Build history of the part. All positions in model axes, mm. Round coordinates to 2 decimals unless told otherwise and drop trailing zeros. Loops run counter-clockwise (first coordinate to the right, second up) from the corner with the lowest first, then second, coordinate; pieces in that order, holes last. Notation, with made-up numbers: (19.25, 83.25) - (54.25, 83.25) arc R13 cw to (54.25, 99.25) - close; hole circle Ø2 at (24.25, 19.5). An arc over 180 degrees is marked (long way). Put each result on its own line as item: value. Start each with the question number.
from build123d import *

# Parameters (mm, degrees)
SKETCH1_W           = 152.4
SKETCH1_H           = 241.3
BOSS_EXTRUDE1_DEPTH = 3.175
SKETCH2_W           = 3.429
SKETCH2_H           = 168.148
SKETCH2_H_2         = 40.386
CUT_EXTRUDE1_DEPTH  = 286.414664348
SKETCH3_W           = 119.38
SKETCH3_H           = 119.38
SKETCH3_W_2         = 74.6125
SKETCH3_H_2         = 25.4
SKETCH3_W_3         = 12.7
SKETCH3_H_3         = 16.256
SKETCH3_W_4         = 5.334
SKETCH3_H_4         = 7.239
CUT_EXTRUDE2_DEPTH  = 286.414664348
SKETCH4_W           = 184.697558878
SKETCH4_H           = 63.754
CUT_EXTRUDE5_DEPTH  = 286.414664348
SKETCH5_W           = 3.429
SKETCH5_H           = 11.43
BOSS_EXTRUDE2_DEPTH = 3.175


with BuildPart() as part:
    # Sketch1 → Boss-Extrude1 (new body)
    with BuildSketch(Plane.XY):
        with Locations((76.2, 120.65)):
            Rectangle(SKETCH1_W, SKETCH1_H)
    extrude(amount=BOSS_EXTRUDE1_DEPTH)

    # Sketch2 → Cut-Extrude1 (cut, through all)
    with BuildSketch(Plane.XY.offset(3.175)):
        with Locations((150.6855, 139.065)):
            Rectangle(SKETCH2_W, SKETCH2_H)
        with Locations((1.7145, 139.065)):
            Rectangle(SKETCH2_W, SKETCH2_H)
        with Locations((150.6855, 20.193)):
            Rectangle(SKETCH2_W, SKETCH2_H_2)
        with Locations((1.7145, 20.193)):
            Rectangle(SKETCH2_W, SKETCH2_H_2)
    extrude(amount=-CUT_EXTRUDE1_DEPTH, mode=Mode.SUBTRACT)

    # Sketch3 → Cut-Extrude2 (cut, through all)
    with BuildSketch(Plane.XY.offset(3.175)):
        Polygon((128.016, 57.15), (140.716, 57.15), (140.716, 44.45), align=None)
        Polygon((125.77093597, 42.20493597), (138.47093597, 42.20493597), (125.77093597, 54.90493597), align=None)
        Polygon((108.966, 57.15), (121.666, 57.15), (121.666, 44.45), align=None)
        Polygon((119.42093597, 42.20493597), (106.72093597, 54.90493597), (106.72093597, 42.20493597), align=None)
        Polygon((89.916, 57.15), (102.616, 57.15), (102.616, 44.45), align=None)
        Polygon((100.37093597, 42.20493597), (87.67093597, 54.90493597), (87.67093597, 42.20493597), align=None)
        Polygon((70.866, 57.15), (83.566, 57.15), (83.566, 44.45), align=None)
        Polygon((81.32093597, 42.20493597), (68.62093597, 54.90493597), (68.62093597, 42.20493597), align=None)
        Polygon((51.816, 57.15), (64.516, 57.15), (64.516, 44.45), align=None)
        Polygon((62.27093597, 42.20493597), (49.57093597, 54.90493597), (49.57093597, 42.20493597), align=None)
        Polygon((32.766, 57.15), (45.466, 57.15), (45.466, 44.45), align=None)
        Polygon((43.22093597, 42.20493597), (30.52093597, 54.90493597), (30.52093597, 42.20493597), align=None)
        Polygon((13.716, 57.15), (26.416, 57.15), (26.416, 44.45), align=None)
        Polygon((24.17093597, 42.20493597), (11.47093597, 54.90493597), (11.47093597, 42.20493597), align=None)
        Polygon((128.016, 38.1), (140.716, 38.1), (140.716, 25.4), align=None)
        with Locations((76.454, 129.159)):
            Rectangle(SKETCH3_W, SKETCH3_H)
        Polygon((125.77093597, 23.15493597), (138.47093597, 23.15493597), (125.77093597, 35.85493597), align=None)
        Polygon((108.966, 38.1), (121.666, 38.1), (121.666, 25.4), align=None)
        Polygon((119.42093597, 23.15493597), (106.72093597, 35.85493597), (106.72093597, 23.15493597), align=None)
        Polygon((89.916, 38.1), (102.616, 38.1), (102.616, 25.4), align=None)
        Polygon((100.37093597, 23.15493597), (87.67093597, 35.85493597), (87.67093597, 23.15493597), align=None)
        Polygon((70.866, 38.1), (83.566, 38.1), (83.566, 25.4), align=None)
        Polygon((81.32093597, 23.15493597), (68.62093597, 35.85493597), (68.62093597, 23.15493597), align=None)
        Polygon((51.816, 38.1), (64.516, 38.1), (64.516, 25.4), align=None)
        Polygon((62.27093597, 23.15493597), (49.57093597, 35.85493597), (49.57093597, 23.15493597), align=None)
        Polygon((32.766, 38.1), (45.466, 38.1), (45.466, 25.4), align=None)
        Polygon((43.22093597, 23.15493597), (30.52093597, 35.85493597), (30.52093597, 23.15493597), align=None)
        Polygon((13.716, 38.1), (26.416, 38.1), (26.416, 25.4), align=None)
        Polygon((24.17093597, 23.15493597), (11.47093597, 35.85493597), (11.47093597, 23.15493597), align=None)
        Polygon((128.016, 19.05), (140.716, 19.05), (140.716, 6.35), align=None)
        Polygon((125.77093597, 4.10493597), (138.47093597, 4.10493597), (125.77093597, 16.80493597), align=None)
        Polygon((108.966, 19.05), (121.666, 19.05), (121.666, 6.35), align=None)
        Polygon((119.42093597, 4.10493597), (106.72093597, 16.80493597), (106.72093597, 4.10493597), align=None)
        Polygon((89.916, 19.05), (102.616, 19.05), (102.616, 6.35), align=None)
        Polygon((100.37093597, 4.10493597), (87.67093597, 16.80493597), (87.67093597, 4.10493597), align=None)
        Polygon((70.866, 19.05), (83.566, 19.05), (83.566, 6.35), align=None)
        Polygon((81.32093597, 4.10493597), (68.62093597, 16.80493597), (68.62093597, 4.10493597), align=None)
        Polygon((51.816, 19.05), (64.516, 19.05), (64.516, 6.35), align=None)
        Polygon((62.27093597, 4.10493597), (49.57093597, 16.80493597), (49.57093597, 4.10493597), align=None)
        Polygon((32.766, 19.05), (45.466, 19.05), (45.466, 6.35), align=None)
        Polygon((43.22093597, 4.10493597), (30.52093597, 16.80493597), (30.52093597, 4.10493597), align=None)
        Polygon((13.716, 19.05), (26.416, 19.05), (26.416, 6.35), align=None)
        Polygon((24.17093597, 4.10493597), (11.47093597, 16.80493597), (11.47093597, 4.10493597), align=None)
        with Locations((54.07025, 215.519)):
            Rectangle(SKETCH3_W_2, SKETCH3_H_2)
        with Locations((129.794, 210.947)):
            Rectangle(SKETCH3_W_3, SKETCH3_H_3)
        with Locations((104.0765, 206.4385)):
            Rectangle(SKETCH3_W_4, SKETCH3_H_4)
    extrude(amount=-CUT_EXTRUDE2_DEPTH, mode=Mode.SUBTRACT)

    # Sketch4 → Cut-Extrude5 (cut, through all)
    with BuildSketch(Plane.XY.offset(3.175)):
        with Locations((77.04209933, 31.877)):
            Rectangle(SKETCH4_W, SKETCH4_H)
    extrude(amount=-CUT_EXTRUDE5_DEPTH, mode=Mode.SUBTRACT)

    # Sketch5 → Boss-Extrude2 (add)
    with BuildSketch(Plane.XY.offset(3.175)):
        with Locations((1.7145, 139.954)):
            Rectangle(SKETCH5_W, SKETCH5_H)
        with Locations((150.6855, 139.954)):
            Rectangle(SKETCH5_W, SKETCH5_H)
    extrude(amount=-BOSS_EXTRUDE2_DEPTH)


solid = part.part
1) Slice it at B-B, the plane y = 138.5. Write the cut outline in (x, z) (3 decimals).
2) Slice it at D-D, the plane y = 208. Write the cut outline in (x, z) (1 decimal).
3) Drop flat-ended pins along their axis: pin 1 Ø1 at (y, z) = (104, 2) entering from -X; pin 2 Ø1.6 at (y, z) = (199, 1.5) entering from +X. Give the stop position or say it passes through.
4) Slice it at C-C, the plane z = 2. State how many separate pieces and enclosed holes the cut face has, and give its area (3 significant figures).
5) Drill centre lines: line 1 (Y direction, x = 70.5, z = 1.35); line 2 (X direction, y = 208.5, z = 0.6); line 3 (Y direction, x = 127, z = 2.2) (3 decimals). Where is each one in solid material? Low to high. Write a range as [from, to].
6) Slice it at A-A, the plane x = 104.5. Write the cut outline in (y, z) (3 decimals), and give its area (3 significant figures).
Taken from the geometry:
1. outline: (0, 0) - (16.764, 0) - (16.764, 3.175) - (0, 3.175) - close; (136.144, 0) - (152.4, 0) - (152.4, 3.175) - (136.144, 3.175) - close
2. outline: (3.4, 0) - (16.8, 0) - (16.8, 3.2) - (3.4, 3.2) - close; (91.4, 0) - (101.4, 0) - (101.4, 3.2) - (91.4, 3.2) - close; (106.7, 0) - (123.4, 0) - (123.4, 3.2) - (106.7, 3.2) - close; (136.1, 0) - (149, 0) - (149, 3.2) - (136.1, 3.2) - close
3. pin 1: stops at x = 3.43
3. pin 2: stops at x = 148.97
4. separate pieces: 1
4. enclosed holes: 4
4. area: 9,650 mm2
5. line 1: y = [63.75, 69.47], [188.85, 202.82], [228.22, 241.3]
5. line 2: x = [3.43, 16.76], [91.38, 101.41], [106.74, 123.44], [136.14, 148.97]
5. line 3: y = [63.754, 69.469], [188.849, 202.819], [219.075, 241.3]
6. outline: (63.754, 0) - (69.469, 0) - (69.469, 3.175) - (63.754, 3.175) - close; (188.849, 0) - (202.819, 0) - (202.819, 3.175) - (188.849, 3.175) - close; (210.058, 0) - (241.3, 0) - (241.3, 3.175) - (210.058, 3.175) - close
6. area: 162 mm2
